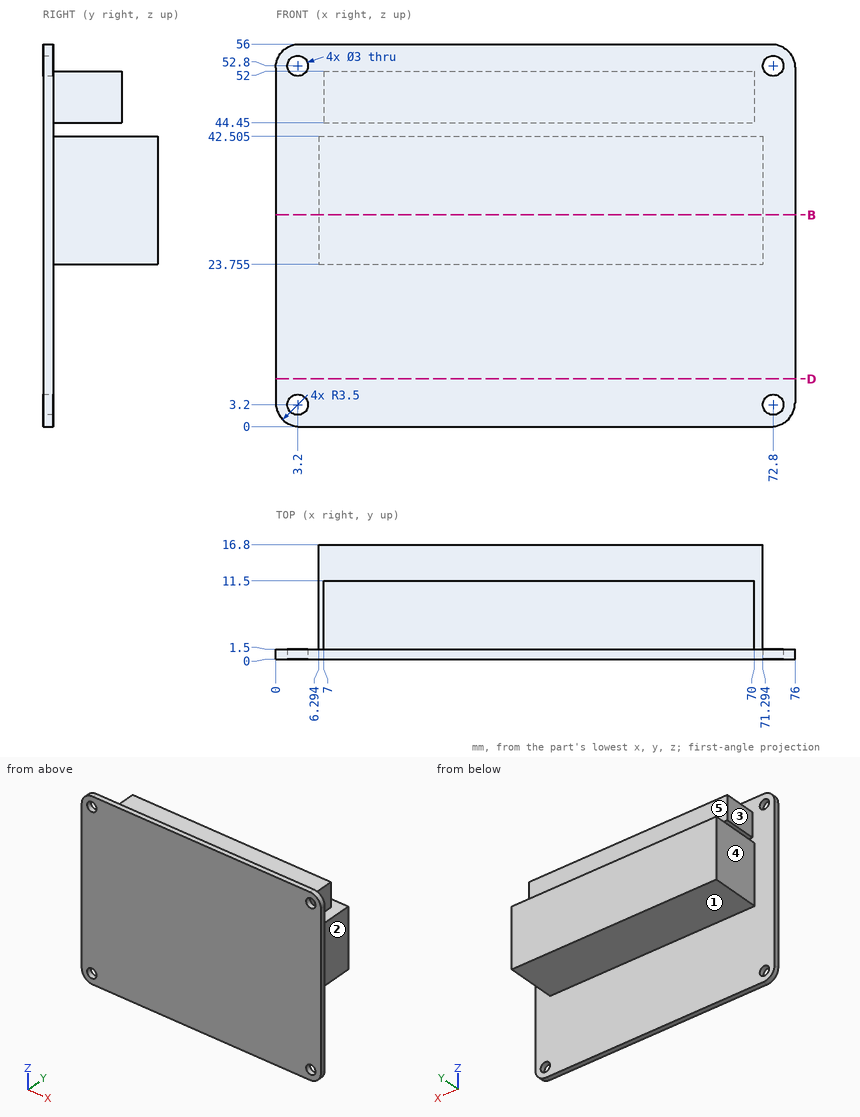
Print and shaded views of the part. All mm, measured from the part's lowest x, y and z. A direction names the side the tool comes from. Round coordinates to 2 decimals unless told otherwise and drop trailing zeros. Write each loop counter-clockwise with the first axis right and the second up, starting at its lowest first coordinate (ties: lowest second). Pieces come first, ordered by that corner, then holes. Notation, with made-up numbers: M 60,-25 L 116,-25 A32 cw 116,7 Z; hole C 75.5,-1.75 d11. An arc over 180 degrees is marked long. One line per question, with ' | ' between items.
(1) Probe line 1 along X through (y, z) = (1.25, 3.2); line 2 along Z through (x, y) = (72.8, 0.7); line 3 along Y through (x, z) = (12, 10). List the from-to ranges inside material, lowest first.
Answer key:
line 1: x = 0.01 to 1.7, 4.7 to 71.3, 74.3 to 75.99 | line 2: z = 0.01 to 1.7, 4.7 to 51.3, 54.3 to 55.99 | line 3: y = 0 to 1.5
(2) Saw through at D-D on z = 7. Write the cut outline in (x, y).
Answer key:
outline: M 0,0 L 76,0 L 76,1.5 L 0,1.5 Z
(3) Saw through at B-B on z = 31. Write the cut outline in (x, y), then the cut area to 3 significant figures.
Answer key:
outline: M 0,0 L 76,0 L 76,1.5 L 71.29,1.5 L 71.29,16.8 L 6.29,16.8 L 6.29,1.5 L 0,1.5 Z | area: 1,110 mm^2
(4) Pin check, flat tips, straight feed: pin 1 (4 mm diameter, centred on x = 63.5, y = 8.5, fed in from +Z); pin 2 (3.5 mm diameter, centred on x = 72.8, z = 52.8, fed in from +Y); pin 3 (8.5 mm diameter, centred on y = 4, z = 49.5, fed in from -X); pin 4 (7.5 mm diameter, centred on y = 8.5, z = 32, fed in from +X). Stop position of each tip, or through.
Answer key:
pin 1: stops at z = 52 | pin 2: stops at y = 1.5 | pin 3: stops at x = 0 | pin 4: stops at x = 71.29
(5) 3-axis set-ups, long thin cutter, end or side, ignore diameter. For the marked faces 1, 2, 3, 4 and 5: which of +Z, -Z, +X, -X, +Y, -Y reach the whole face in a straight line?
Answer key:
face 1: -Z, +X, -X, +Y | face 2: +Z, -Z, +X, +Y | face 3: +Z, -X, +Y | face 4: +Z, -Z, -X, +Y | face 5: +Z, +X, -X, +Y
